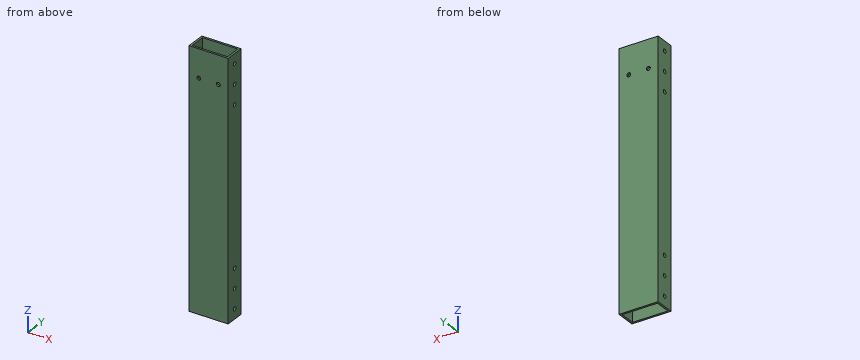
Autodesk Inventor part; units mm, degrees
ref_plane "YZ Plane" through (0, 0, 0) normal (1, 0, 0) x (0, 1, 0)
ref_plane "XZ Plane" through (0, 0, 0) normal (0, 1, 0) x (-1, 0, 0)
ref_plane "XY Plane" through (0, 0, 0) normal (0, 0, 1) x (1, 0, 0)
sketch "Sketch1" plane through (0, 0, 0) normal (0, 0, 1) x (1, 0, 0)
  line L0 (0, 0) -> (-50.8, 0)
  line L1 (-50.8, 0) -> (-50.8, 25.4)
  line L2 (-50.8, 25.4) -> (0, 25.4)
  line L3 (0, 25.4) -> (0, 0)
  line L4 (-48.26, 22.86) -> (-2.54, 22.86)
  line L5 (-2.54, 22.86) -> (-2.54, 2.54)
  line L6 (-2.54, 2.54) -> (-48.26, 2.54)
  line L7 (-48.26, 2.54) -> (-48.26, 22.86)
  dimension "d0" = 25.4
  dimension "d1" = 50.8
  dimension "d2" = 2.54
  dimension "d3" = 2.54
  dimension "d4" = 2.54
  dimension "d5" = 2.54
extrude "Extrusion1" add sketch "Sketch1" along normal blind 330.2
sketch "Sketch2" plane through (-50.8, 0, 0) normal (-1, 0, 0) x (0, 0, 1)
  circle A0 centre (12.7, 12.7) radius 2.5797
  circle A1 centre (38.1, 12.7) radius 2.5797
  circle A2 centre (63.5, 12.7) radius 2.5797
  circle A3 centre (266.7, 12.7) radius 2.5797
  circle A4 centre (292.1, 12.7) radius 2.5797
  circle A5 centre (317.5, 12.7) radius 2.5797
  line L0 (0, 0) -> (0, 25.4)
  line L1 (330.2, 25.4) -> (330.2, 0)
  line L2 (0, 25.4) -> (330.2, 25.4)
  dimension "d8" = 12.7
  dimension "d9" = 25.4
  dimension "d10" = 25.4
  dimension "d11" = 25.4
  dimension "d12" = 25.4
  dimension "d13" = 12.7
  dimension "d14" = 5.1594
  dimension "d15" = 5.1594
  dimension "d16" = 5.1594
  dimension "d19" = 5.1594
  dimension "d20" = 5.1594
  dimension "d21" = 5.1594
  dimension "d22" = 12.7
  dimension "d23" = 12.7
  dimension "d24" = 12.7
  dimension "d25" = 12.7
  dimension "d26" = 12.7
  dimension "d27" = 12.7
extrude "Extrusion2" cut sketch "Sketch2" against normal blind 279.4
sketch "Sketch3" plane through (-50.8, 0, 0) normal (0, -1, 0) x (1, 0, 0)
  circle A0 centre (12.7, 293.8134) radius 2.5797
  circle A1 centre (38.1, 293.8134) radius 2.5797
  line L0 (0, 0) -> (0, 330.2)
  point P0 (50.8, 0)
  dimension "d30" = 5.1594
  dimension "d31" = 5.1594
  dimension "d32" = 12.7
  dimension "d33" = 25.4
extrude "Extrusion3" cut sketch "Sketch3" against normal blind 279.4
equation "\"d10\" = d9"
equation "\"d11\" = d9"
equation "\"d15\" = d14"
equation "\"d16\" = d14"
equation "\"d19\" = d14"
equation "\"d20\" = d14"
equation "\"d21\" = d14"
equation "\"d26\" = d25"
equation "\"d27\" = d25"
equation "\"d31\" = d30"
properties part number "ATACHMENT BAR"
Check sheet for the modelled part. Datum: model origin and axes. Units: mm. Round coordinates to 2 decimals unless told otherwise and drop trailing zeros. Loops run counter-clockwise (first coordinate to the right, second up) from the corner with the lowest first, then second, coordinate; pieces in that order, holes last. Notation, with made-up numbers: (1.25, 8) - (14.25, 8) arc R9 ccw to (14.25, 21) - close; hole circle Ø9 at (76, -23). An arc over 180 degrees is marked (long way). Write item = value, one per line. Start each with the question number.
Q1. Section check B-B (x = -22). Record the boundary of the cut face in (y, z).
Q2. Section check C-C (z = 120). Record the boundary of the cut face in (x, y).
Q3. Depth check by flat-ended pin: P1, Ø12, axis at x = -32, y = 11.5, coming from the +Z side. Enter the tip coordinate at first touch or a pass-through.
Q4. Section check A-A (y = 6). Record the boundary of the cut face in (x, z), plus the area to 3 significant figures.
Q5. Thickness scan on L1, parallel to Y at x = -28.5, z = 269; L2, parallel to X at y = 9.5, z = 89; L3, parallel to Y at x = -1.2, z = 317.5. Record the ranges inside material, lowest first.
Derived:
q1.outline = (0, 0) - (2.54, 0) - (2.54, 330.2) - (0, 330.2) - close; (22.86, 0) - (25.4, 0) - (25.4, 330.2) - (22.86, 330.2) - close
q2.outline = (-50.8, 0) - (0, 0) - (0, 25.4) - (-50.8, 25.4) - close; hole (-48.26, 2.54) - (-2.54, 2.54) - (-2.54, 22.86) - (-48.26, 22.86) - close
q3.P1 = through
q4.outline = (-50.8, 0) - (-48.26, 0) - (-48.26, 330.2) - (-50.8, 330.2) - close; (-2.54, 0) - (0, 0) - (0, 330.2) - (-2.54, 330.2) - close
q4.area = 1,680 mm^2
q5.L1 = 0 to 2.54, 22.86 to 25.4
q5.L2 = -50.8 to -48.26, -2.54 to 0
q5.L3 = 0 to 10.12, 15.28 to 25.4
